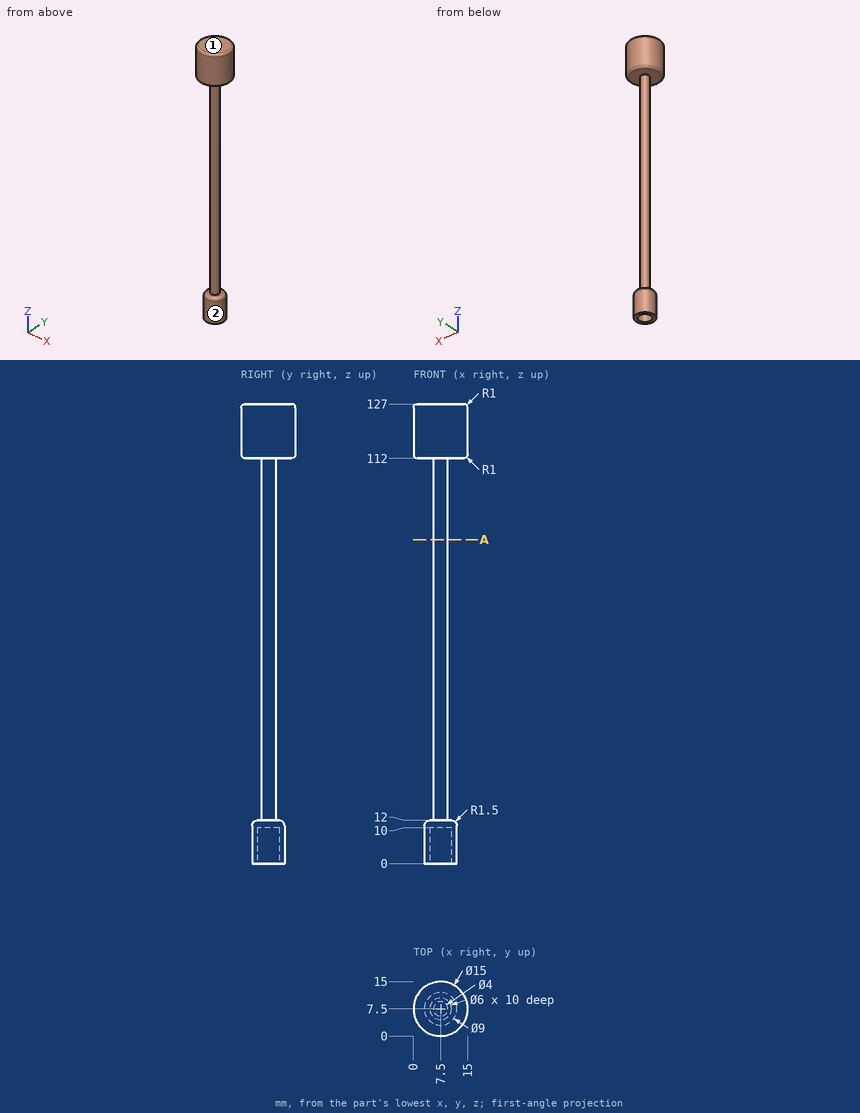
Input: dimensioned drawing with shaded views. Units: mm. Origin: part minimum x, y, z. A direction names the side the tool comes from. Give positions to 0.01 mm unless a question says otherwise; leave off trailing zeros. Order: outer loops, then holes, each group sorted by start corner. A loop starts at its lowest first (then second) coordinate and runs counter-clockwise, first axis right, second up. Notation, with made-up numbers: (36, 32.5) -> (46, 32.5) arc R19 cw to (46, 51.5) -> close; hole circle Ø5 at (81.5, -37). An arc over 180 degrees is marked (long way). Write item = value, one per line.
Item 1: Section query A-A (z = 89.5). Output: boundary loops of the cut face in (x, y), then the cut area to 3 significant figures.
Check result:
outline = circle Ø4 at (7.5, 7.5)
area = 12.6 mm²
Item 2: Contact query for flat-ended pins moving along their axis: pin 1 (5 mm diameter, centred on x = 9, z = 36, fed in from +Y); pin 2 (5 mm diameter, centred on x = 6.5, y = 8, fed in from -Z); pin 3 (5 mm diameter, centred on x = 4.5, z = 101, fed in from +Y); pin 4 (5 mm diameter, centred on x = 8, z = 43, fed in from -Y). Output: stop coordinate, or through.
Check result:
pin_1 = 9.5
pin_2 = 0
pin_3 = 9.44
pin_4 = 5.5
Item 3: Ray query, probe 1 along Y at (x, z) = (7.5, 5.75); probe 2 along Z at (x, y) = (7.5, 5); probe 3 along Z at (x, y) = (11.75, 5.75). Return the intervals inside material, ascending.
Check result:
probe_1 = 3 to 4.5, 10.5 to 12
probe_2 = 10 to 12, 112 to 127
probe_3 = 112 to 127
Item 4: Set-up query: the marked faces 1 and 2. Return all of +Z, -Z, +X, -X, +Y, -Y with unobstructed straight access to the full face (end or side cutting, diameter ignored); none if empty.
Check result:
face_1 = +Z, +X, -X, +Y, -Y
face_2 = -Z
